Autodesk Inventor part; units mm, degrees
ref_plane "YZ Plane" through (0, 0, 0) normal (1, 0, 0) x (0, 1, 0)
ref_plane "XZ Plane" through (0, 0, 0) normal (0, 1, 0) x (-1, 0, 0)
ref_plane "XY Plane" through (0, 0, 0) normal (0, 0, 1) x (1, 0, 0)
sketch "Skizze1" plane through (0, 0, 0) normal (0, 1, 0) x (-1, 0, 0)
  line L0 (12.5, -75) -> (-12.5, -75)
  line L1 (-12.5, -75) -> (-12.5, 75)
  line L2 (-12.5, 75) -> (12.5, 75)
  line L3 (12.5, 75) -> (12.5, -75)
  line L4 (12.5, -75) -> (-12.5, 75) construction
  line L5 (12.5, 75) -> (-12.5, -75) construction
  line L6 (7.5, -75) -> (-7.5, -75)
  line L7 (-7.5, -75) -> (-7.5, -80)
  line L8 (-7.5, -80) -> (7.5, -80)
  line L9 (7.5, -80) -> (7.5, -75)
  line L10 (7.5, 75) -> (-7.5, 75)
  line L11 (-7.5, 75) -> (-7.5, 80)
  line L12 (-7.5, 80) -> (7.5, 80)
  line L13 (7.5, 80) -> (7.5, 75)
  line L14 (12.5, -1) -> (10.5, -1)
  line L15 (12.5, 1) -> (10.5, 1)
  line L16 (-12.5, -1) -> (-10.5, -1)
  line L17 (-12.5, 1) -> (-10.5, 1)
  arc A0 (10.5, 1) -> (10.5, -1) centre (10.5, 0) ccw
  arc A1 (-10.5, -1) -> (-10.5, 1) centre (-10.5, 0) ccw
  point P0 (0, 0)
  point P1 (0, 0)
  point P2 (7.5, -77.5)
  point P3 (0, 0)
  point P4 (-7.5, 75)
  point P5 (-7.5, -75)
  dimension "d0" = 150
  dimension "d1" = 5
  dimension "d2" = 5
  dimension "d3" = 5
  dimension "d4" = 15
  dimension "d5" = 2
  dimension "d6" = 2
  dimension "d7" = 1
extrude "Extrusion1" add sketch "Skizze1" along normal blind 5 contours L0 L1 L16 A1 L17 L2 L3 L15 A0 L14 | L9 L8 L7 L0 | L2 L11 L12 L13
equation "\"t\" = 15"
properties part number "Verbinder_t80"
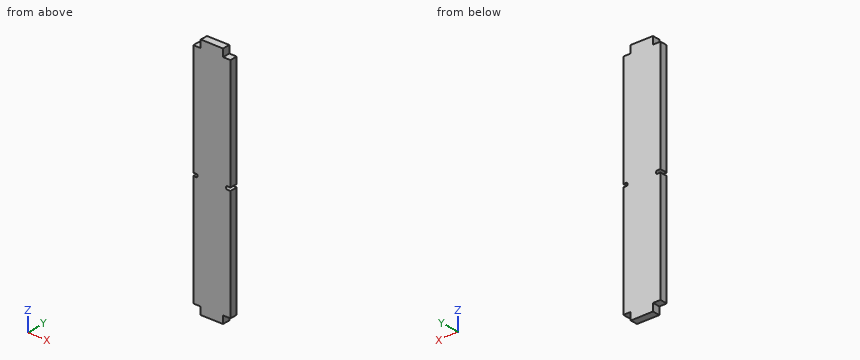
Design review of the part built by this model. Coordinates are the model's own, in mm. Coordinates: 2 decimals unless noted, no trailing zeros. Loops run counter-clockwise (first coordinate to the right, second up) from the corner with the lowest first, then second, coordinate; pieces in that order, holes last.
Q1. To check wall thickness, follow line 1 (Z direction, x = 11.25, y = 1.8); line 2 (Z direction, x = -9, y = 3.6). State the ranges of each line that lie inside material, in increasing order.
Reported:
line 1: z = -75 to -1, 1 to 75
line 2: z = -75 to 75
Q2. We need section A-A on y = 4.1. State the section outline as (x, z) points.
Reported:
outline: (-12.5, -75) - (-7.5, -75) - (-7.5, -80) - (7.5, -80) - (7.5, -75) - (12.5, -75) - (12.5, -1) - (10.5, -1) arc R1 cw to (10.5, 1) - (12.5, 1) - (12.5, 75) - (7.5, 75) - (7.5, 80) - (-7.5, 80) - (-7.5, 75) - (-12.5, 75) - (-12.5, 1) - (-10.5, 1) arc R1 cw to (-10.5, -1) - (-12.5, -1) - close
Q3. For pin 1 (2.5 mm diameter, centred on x = 10, y = 3.5, fed in from -Z); pin 2 (1.5 mm diameter, centred on y = 3, z = -77, fed in from -X); pin 3 (1 mm diameter, centred on x = -12, y = 3.5, fed in from +Z), all flat-tipped, find the tip position at first contact; note any pin that passes through.
Reported:
pin 1: stops at z = -75
pin 2: stops at x = -7.5
pin 3: stops at z = 75
